Geometry check sheet. Reference: the model listing, model coordinates, mm. Face numbers are marked on the shaded views. Round coordinates to 2 decimals unless told otherwise and drop trailing zeros. Write each loop counter-clockwise with the first axis right and the second up, starting at its lowest first coordinate (ties: lowest second). Pieces come first, ordered by that corner, then holes. Notation, with made-up numbers: (70, -37.5) -> (81, -37.5) arc R7 ccw to (81, -28.5) -> close; hole circle Ø1 at (9, 87.5). An arc over 180 degrees is marked (long way). Put each result on its own line as item: value. Start each with the question number.
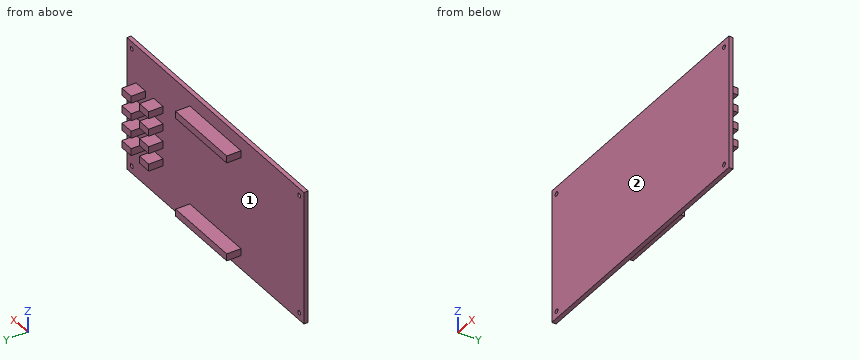
from build123d import *

# Parameters (mm, degrees)
ESQUISSE1_W      = 190.5
ESQUISSE1_H      = 94
ESQUISSE1_R      = 1.5
EXTRUSION1_DEPTH = 3
ESQUISSE2_W      = 55
ESQUISSE2_H      = 5
EXTRUSION2_DEPTH = 10
ESQUISSE4_W      = 10
ESQUISSE4_H      = 5
EXTRUSION4_DEPTH = 10


with BuildPart() as part:
    # Esquisse1 → Extrusion1 (new body)
    with BuildSketch(Plane(origin=(0, 0, 0), x_dir=(1, 0, 0), z_dir=(0, 1, 0))):
        with Locations((95.25, 47)):
            Rectangle(ESQUISSE1_W, ESQUISSE1_H)
        with Locations((5.08, 88.92)):
            Circle(ESQUISSE1_R, mode=Mode.SUBTRACT)
        with Locations((185.42, 88.92)):
            Circle(ESQUISSE1_R, mode=Mode.SUBTRACT)
        with Locations((185.42, 5.08)):
            Circle(ESQUISSE1_R, mode=Mode.SUBTRACT)
        with Locations((5.08, 5.08)):
            Circle(ESQUISSE1_R, mode=Mode.SUBTRACT)
    extrude(amount=EXTRUSION1_DEPTH)

    # Esquisse2 → Extrusion2 (add)
    with BuildSketch(Plane(origin=(0, 3, 0), x_dir=(1, 0, 0), z_dir=(0, 1, 0))):
        with Locations((95.25, 82)):
            Rectangle(ESQUISSE2_W, ESQUISSE2_H)
        with Locations((95.25, 12)):
            Rectangle(ESQUISSE2_W, ESQUISSE2_H)
    extrude(amount=EXTRUSION2_DEPTH)

    # Esquisse4 → Extrusion4 (add)
    with BuildSketch(Plane(origin=(0, 3, 0), x_dir=(1, 0, 0), z_dir=(0, 1, 0))):
        with Locations((175.67625178, 66.658495743)):
            Rectangle(ESQUISSE4_W, ESQUISSE4_H)
        with Locations((156.685730764, 66.658495743)):
            Rectangle(ESQUISSE4_W, ESQUISSE4_H)
        with Locations((156.685730764, 41.658495743)):
            Rectangle(ESQUISSE4_W, ESQUISSE4_H)
        with Locations((156.685730764, 29.158495743)):
            Rectangle(ESQUISSE4_W, ESQUISSE4_H)
        with Locations((156.685730764, 54.158495743)):
            Rectangle(ESQUISSE4_W, ESQUISSE4_H)
        with Locations((175.67625178, 41.658495743)):
            Rectangle(ESQUISSE4_W, ESQUISSE4_H)
        with Locations((175.67625178, 29.158495743)):
            Rectangle(ESQUISSE4_W, ESQUISSE4_H)
        with Locations((175.67625178, 54.158495743)):
            Rectangle(ESQUISSE4_W, ESQUISSE4_H)
    extrude(amount=EXTRUSION4_DEPTH)


solid = part.part
(1) Sectioned sample at B-B (y = 10.5). State how many separate pieces and enclosed holes the cut face has, and give its area (3 significant figures).
(2) Go/stop test with flat-tipped pins: pin 1 Ø2.5 at (y, z) = (6, -53) entering from -X; pin 2 Ø4 at (y, z) = (10.5, -81.5) entering from -X; pin 3 Ø1.5 at (y, z) = (9, -28.5) entering from +X. Record where each tip stops, or that it passes through.
(3) Mould release check, pull along Z, two halves, no side actions. Record for the marked faces 1 and 2: +Z half, -Z half, draft (parallel to the pull), parting line (faces both ways), or undercut.
(4) Material ranges on L1, parallel to Z at x = 161, y = 9.5; L2, parallel to X at y = 1.6, z = -5.08; L3, parallel to Z at x = 185.42, y = 1.7, recorded low to high. Write a range as from..to.
(5) Sectioned sample at A-A (z = -46). Record the cut outline in (x, y), and give its area (4 significant figures).
(6) Sectioned sample at C-C (x = 42.5). Record the cut outline in (y, z), and give its area (3 significant figures).
Found:
1. separate pieces: 10
1. enclosed holes: 0
1. area: 950 mm2
2. pin 1: x = 151.69
2. pin 2: x = 67.75
2. pin 3: x = 180.68
3. face 1: undercut
3. face 2: draft
4. L1: -69.16..-64.16, -56.66..-51.66, -44.16..-39.16, -31.66..-26.66
4. L2: 0..3.58, 6.58..183.92, 186.92..190.5
4. L3: -94..-90.42, -87.42..-6.58, -3.58..0
5. outline: (0, 0) -> (190.5, 0) -> (190.5, 3) -> (0, 3) -> close
5. area: 571.5 mm2
6. outline: (0, -94) -> (3, -94) -> (3, 0) -> (0, 0) -> close
6. area: 282 mm2
